The listing builds one solid part. Answer for the finished solid, in the listing's coordinates (mm). Face numbers are marked on the shaded views. Give positions to 0.01 mm unless a question says otherwise; leave off trailing zeros. Order: outer loops, then holes, each group sorted by start corner. A loop starts at its lowest first (then second) coordinate and runs counter-clockwise, first axis right, second up. Notation, with made-up numbers: (8.25, 89.25) - (31.25, 89.25) arc R16 cw to (31.25, 115.25) - close; hole circle Ø1 at (-24, 80.25). An arc over 180 degrees is marked (long way). Use a Markdown table: item, result. Add a question column.
1) The mould has two halves that part along Y. Classify the marked faces 1 and 2: released by +Y, released by -Y, zero draft, split by the parting line, or undercut.
2) Find section C-C, the plane z = 413. Determine the outline of the cut face in (x, y), plus the area to 3 significant figures.
3) Straight lines are drawn through the part: line 1 (Y direction, x = 0, z = 614); line 2 (Y direction, x = 4, z = 420). For each, find the intervals that lie inside material, in ascending order.
4) Find section B-B, the plane x = 29. Determine the outline of the cut face in (y, z).
5) Find section A-A, the plane y = 17.5. Determine the outline of the cut face in (x, z).
6) Flat-ended cylindrical pins translate along their axes: pin 1 (4 mm diameter, centred on x = -10.5, z = 542.5, fed in from +Y); pin 2 (4 mm diameter, centred on x = 3, z = 587.5, fed in from +Y); pin 3 (1 mm diameter, centred on x = 24.5, z = 221, fed in from -Y); pin 4 (10 mm diameter, centred on x = -27, y = 0, fed in from +Z). Find the tip coordinate at first contact, or state that the pin passes through.
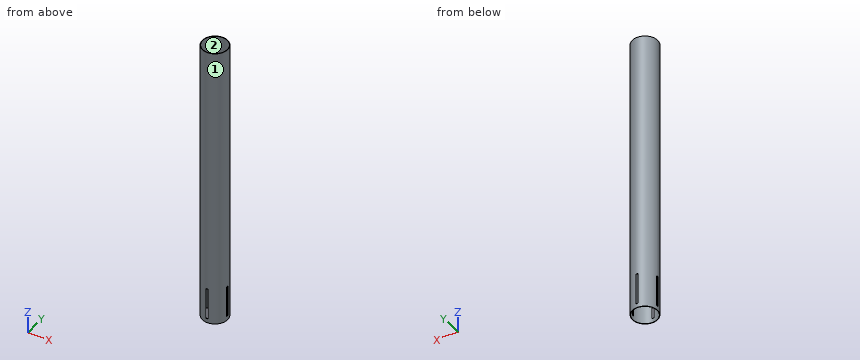
Autodesk Inventor part; units mm, degrees
ref_plane "YZ Plane" through (0, 0, 0) normal (1, 0, 0) x (0, 1, 0)
ref_plane "XZ Plane" through (0, 0, 0) normal (0, 1, 0) x (-1, 0, 0)
ref_plane "XY Plane" through (0, 0, 0) normal (0, 0, 1) x (1, 0, 0)
sketch "Sketch1" plane through (0, 0, 0) normal (1, 0, 0) x (0, 1, 0)
  line L0 (0, 0) -> (-38.1, 0)
  line L1 (-38.1, 0) -> (-38.1, 864)
  line L2 (-38.1, 864) -> (0, 864)
  line L3 (0, 864) -> (0, 0)
  dimension "d0" = 38.1
  dimension "d1" = 864
revolve "Revolution1" add sketch "Sketch1" angle 360 about axis through (0, 0, 864) along (0, 0, -1)
sketch "Sketch2" plane through (0, 0, 864) normal (0, 0, 1) x (1, 0, 0)
  circle A0 centre (0, 0) radius 36.83
  circle A1 centre (0, 0) radius 38.1
  dimension "d3" = 1.27
extrude "Extrusion1" cut sketch "Sketch2" against normal through all contours A0
sketch "Sketch3" plane through (0, 0, 0) normal (1, 0, 0) x (0, 1, 0)
  line L0 (0, 0) -> (0, 12.7)
  line L1 (0, 12.7) -> (3.175, 12.7)
  line L2 (3.175, 12.7) -> (3.175, 107.95)
  line L3 (3.175, 107.95) -> (0, 107.95)
  line L4 (0, 12.7) -> (-3.175, 12.7)
  line L5 (-3.175, 12.7) -> (-3.175, 107.95)
  line L6 (-3.175, 107.95) -> (0, 107.95)
  dimension "d6" = 12.7
  dimension "d10" = 3.175
  dimension "d11" = 95.25
  dimension "d12" = 3.175
extrude "Extrusion2" cut sketch "Sketch3" along normal through all both and the other way through all
sketch "Sketch4" plane through (0, 0, 0) normal (0, 1, 0) x (-1, 0, 0)
  line L0 (0, 0) -> (0, 12.7)
  line L1 (0, 12.7) -> (3.175, 12.7)
  line L2 (3.175, 12.7) -> (3.175, 107.95)
  line L3 (3.175, 107.95) -> (0, 107.95)
  line L4 (0, 12.7) -> (-3.175, 12.7)
  line L5 (-3.175, 12.7) -> (-3.175, 107.95)
  line L6 (-3.175, 107.95) -> (0, 107.95)
  dimension "d15" = 12.7
  dimension "d16" = 3.175
  dimension "d17" = 95.25
  dimension "d18" = 3.175
  dimension "d19" = 95.25
extrude "Extrusion3" cut sketch "Sketch4" along normal through all both and the other way through all
properties part number "Body Tube"
The answers:
| question | item | result |
|---|---|---|
| 1 | face 1 | split by the parting line |
| 1 | face 2 | undercut |
| 2 | outline | circle Ø76.2 at (0, 0); hole circle Ø73.66 at (0, 0) |
| 2 | area | 299 mm2 |
| 3 | line 1 | -38.1 to -36.83, 36.83 to 38.1 |
| 3 | line 2 | -37.89 to -36.61, 36.61 to 37.89 |
| 4 | outline | (-24.71, 0) - (-22.7, 0) - (-22.7, 864) - (-24.71, 864) - close; (22.7, 0) - (24.71, 0) - (24.71, 864) - (22.7, 864) - close |
| 5 | outline | (-33.84, 0) - (-32.41, 0) - (-32.41, 864) - (-33.84, 864) - close; (32.41, 0) - (33.84, 0) - (33.84, 864) - (32.41, 864) - close |
| 6 | pin 1 | y = 37.14 |
| 6 | pin 2 | y = 38.09 |
| 6 | pin 3 | y = -29.59 |
| 6 | pin 4 | through |
